Geometry check sheet. Reference: drawing and pictorial views, mm from the part's lowest x, y, z. A direction names the side the tool comes from. Give positions to 0.01 mm unless a question says otherwise; leave off trailing zeros. Order: outer loops, then holes, each group sorted by start corner. A loop starts at its lowest first (then second) coordinate and runs counter-clockwise, first axis right, second up. Notation, with made-up numbers: (-1.5, 8) -> (51.5, 8) arc R16 cw to (51.5, 30) -> close; hole circle Ø8 at (84, -36.75). An arc over 180 degrees is marked (long way). Write each question's results on one line, items separated by ' | '. Start each with the question number.
1. Cross-section at B-B, the plane z = 9.05. Enter the section's corners in (x, y) (1 decimal).
2. Cross-section at D-D, the plane x = 15.5. Enter the section's corners in (y, z).
3. Cross-section at A-A, the plane x = 2.5. Enter the section's corners in (y, z) (1 decimal).
4. Cross-section at C-C, the plane y = 3.75. Enter the section's corners in (x, z).
5. Mould release check, pull along X, two halves, no side actions. Record for the marked faces 6, 7 and 8: +X half, -X half, draft (parallel to the pull), parting line (faces both ways), or undercut.
6. Material ranges on L1, parallel to X at y = 17.6, z = 9.05; L2, parallel to X at y = 24.5, z = 9.05 (1 decimal); L3, parallel to Y at x = 28.5, z = 11, recorded low to high. Write a range as from..to.
7. Depth check by flat-ended pin: pin 1 Ø2.5 at (x, z) = (30.2, 9.05) entering from +Y; pin 2 Ø2 at (y, z) = (17.5, 1.5) entering from -X; pin 3 Ø6 at (x, z) = (11.5, 6.5) entering from +Y; pin 4 Ø4 at (x, z) = (31, 12) entering from -Y. Enter the tip coordinate at first touch or a pass-through.
8. Set-up check for the marked faces 1, 2, 3, 4 and 5: record each of +Z, -Z, +X, -X, +Y, -Y from which the full face is reachable in a straight line by a thin tool's end or side.
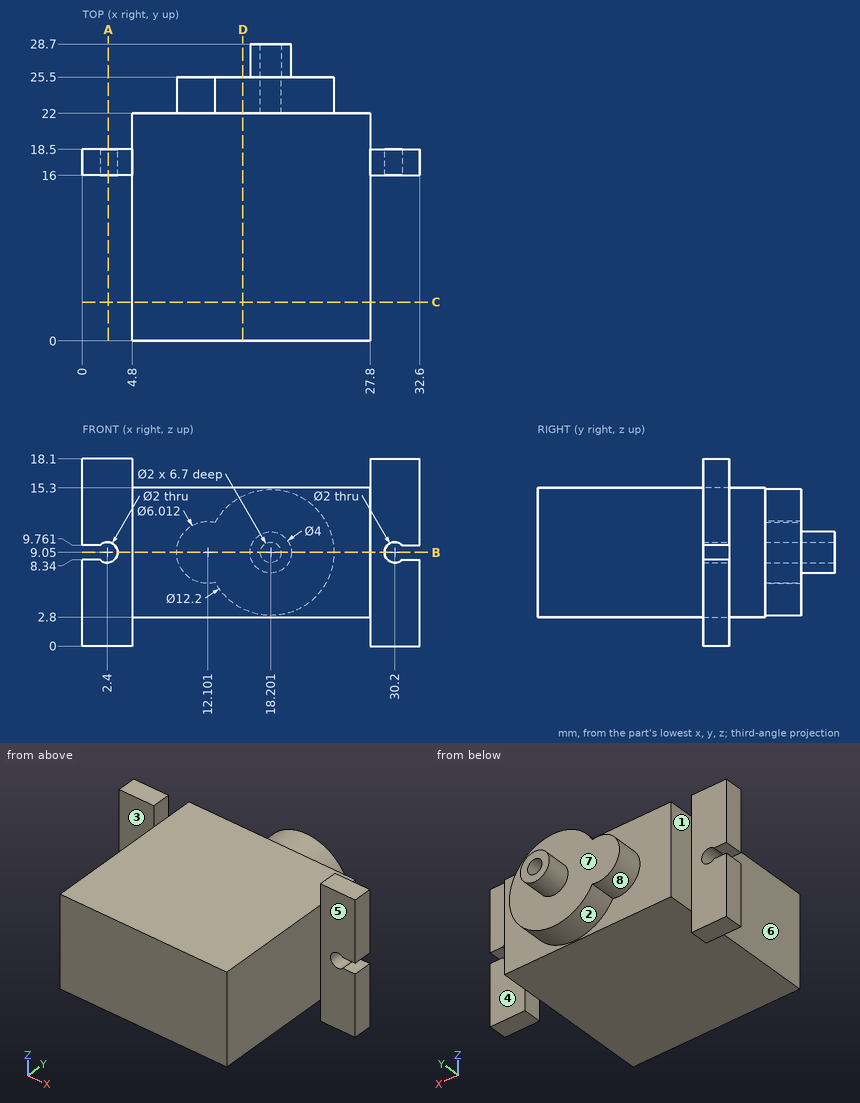
Results below:
1) outline: (3.4, 16) -> (4.8, 16) -> (4.8, 0) -> (27.8, 0) -> (27.8, 16) -> (29.2, 16) -> (29.2, 18.5) -> (27.8, 18.5) -> (27.8, 22) -> (24.3, 22) -> (24.3, 25.5) -> (20.2, 25.5) -> (20.2, 28.7) -> (19.2, 28.7) -> (19.2, 22) -> (17.2, 22) -> (17.2, 28.7) -> (16.2, 28.7) -> (16.2, 25.5) -> (9.1, 25.5) -> (9.1, 22) -> (4.8, 22) -> (4.8, 18.5) -> (3.4, 18.5) -> close
2) outline: (0, 2.8) -> (22, 2.8) -> (22, 3.58) -> (25.5, 3.58) -> (25.5, 14.52) -> (22, 14.52) -> (22, 15.3) -> (0, 15.3) -> close
3) outline: (16, 0) -> (18.5, 0) -> (18.5, 8.1) -> (16, 8.1) -> close; (16, 10) -> (18.5, 10) -> (18.5, 18.1) -> (16, 18.1) -> close
4) outline: (4.8, 2.8) -> (27.8, 2.8) -> (27.8, 15.3) -> (4.8, 15.3) -> close
5) face 6: -X half | face 7: draft | face 8: undercut
6) L1: x = 3.4..29.2 | L2: x = 9.1..17.2, 19.2..24.3 | L3: y = 16..18.5
7) pin 1: stops at y = 18.5 | pin 2: stops at x = 0 | pin 3: stops at y = 25.5 | pin 4: stops at y = 16
8) face 1: +Z, -Z, -X, +Y | face 2: +Y | face 3: +Z, -Z, -X, -Y | face 4: +Z, -Z, +X, +Y | face 5: +Z, -Z, +X, -Y
